Design review of the part built by this model. Coordinates are the model's own, in mm. Give positions to 0.01 mm unless a question says otherwise; leave off trailing zeros. Loops run counter-clockwise (first coordinate to the right, second up) from the corner with the lowest first, then second, coordinate; pieces in that order, holes last. Notation, with made-up numbers: (53, 46) -> (68, 46) arc R31 ccw to (68, 81) -> close; hole circle Ø10 at (32, 23.25). An arc over 180 degrees is marked (long way). Answer as CSV lines item,"result".
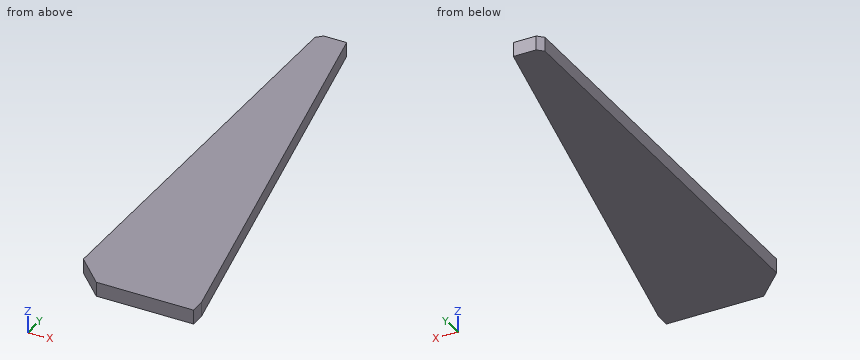
from build123d import *

# Parameters (mm, degrees)
EXTRUDE_1_DEPTH = 2.5
CHAMFER_1_SIZE  = 10
CHAMFER_2_SIZE  = 2


with BuildPart() as part:
    # Эскиз1 → Бобышка-Вытянуть1 (new, symmetric)
    with BuildSketch(Plane.XY):
        Polygon((0, 0), (0, 160), (10, 160), (44, 5), (44, 0), align=None)
    extrude(amount=EXTRUDE_1_DEPTH, both=True)

    # Фаска1
    chamfer_1_edges = [part.edges().sort_by_distance(p)[0] for p in [
        (0, 0, 0),
    ]]
    chamfer(chamfer_1_edges, length=CHAMFER_1_SIZE)

    # Фаска2
    chamfer_2_edges = [part.edges().sort_by_distance(p)[0] for p in [
        (0, 160, 0),
    ]]
    chamfer(chamfer_2_edges, length=CHAMFER_2_SIZE)


solid = part.part
Q1. We need section C-C, the plane y = 147.5. State the section outline as (x, z) points.
Filled sheet:
outline,"(0, -2.5) -> (12.74, -2.5) -> (12.74, 2.5) -> (0, 2.5) -> close"
Q2. We need section A-A, the plane z = -0.8. State the section outline as (x, y) points, and give its area (3 significant figures).
Filled sheet:
outline,"(0, 10) -> (10, 0) -> (44, 0) -> (44, 5) -> (10, 160) -> (2, 160) -> (0, 158) -> close"
area,"4,350 mm^2"
Q3. Clearance check with flat-ended pins moving along their axes: pin 1 Ø6 at (x, y) = (26.5, 110) entering from -Z; pin 2 Ø12 at (x, y) = (23.5, 118) entering from -Z. State where each tip first meets the part, or that it passes through.
Filled sheet:
pin 1,"passes through"
pin 2,"stops at z = -2.5"
Q4. We need section B-B, the plane x = 5. State the section outline as (y, z) points, and give its area (3 significant figures).
Filled sheet:
outline,"(5, -2.5) -> (160, -2.5) -> (160, 2.5) -> (5, 2.5) -> close"
area,"775 mm^2"
Q5. To check wall thickness, follow probe 1 along Y at (x, z) = (5, 1.45); probe 2 along X at (y, z) = (24.5, 0.45); probe 3 along X at (y, z) = (85.5, -1). State the ranges of each line that lie inside material, in increasing order. Write a range as from..to.
Filled sheet:
probe 1,"y = 5..160"
probe 2,"x = 0..39.72"
probe 3,"x = 0..26.34"
